Read the model definition and answer for the solid it produces. Units are mm, in the model's axes. Round coordinates to 2 decimals unless told otherwise and drop trailing zeros. Order: outer loops, then holes, each group sorted by start corner. A loop starts at its lowest first (then second) coordinate and runs counter-clockwise, first axis right, second up. Notation, with made-up numbers: (73, 83) - (118, 83) arc R17 ccw to (118, 116) - close; hole circle Ø1 at (43, 25). An arc over 180 degrees is marked (long way). Answer as a JSON object with one key per item and string values. Group by question number.
Q1. Consider line 1 (Y direction, x = 62, z = 1.05); line 2 (X direction, y = -14.75, z = 1.15); line 3 (Y direction, x = 254, z = 0.2). Determine where each line is inside the solid, lowest interval first.
Q2. Given pin 1 Ø4.5 at (x, y) = (254, -13) entering from +Z, flat-ended and moving along its own axis, determine where the tip first touches the part or whether it passes through.
Q3. A cutting plane is placed at A-A on x = 187.5. Determine the outline of the cut face in (y, z) (3 decimals), and give its area (3 significant figures).
Q4. A cutting plane is placed at B-B on z = 1.55. Count the separate pieces of the cut face and the enclosed holes in it, and give its area (3 significant figures).
Autodesk Fusion 360 part; units mm, degrees
sketch "Sketch1" plane through (0, 0, 0) normal (0, 0, 1) x (1, 0, 0)
  line L0 (0, 0) -> (0, -12.7)
  line L1 (12.7, 0) -> (254, 0)
  line L2 (254, -25.4) -> (12.7, -25.4)
  line L3 (0, -25.4) -> (0, -12.7)
  arc A0 (12.7, 0) -> (0, -12.7) centre (12.7, -12.7) ccw
  arc A1 (0, -12.7) -> (12.7, -25.4) centre (12.7, -12.7) ccw
  circle A2 centre (254, -12.7) radius 1.27
  line L4 (254, -25.4) -> (255.27, -25.4)
  line L5 (255.27, 0) -> (254, 0)
  line L6 (255.27, 0) -> (245.11, 0)
  line L7 (245.11, -25.4) -> (255.27, -25.4)
  arc A3 (257.81, -12.7) -> (245.11, 0) centre (245.11, -12.7) ccw
  arc A4 (245.11, -25.4) -> (257.81, -12.7) centre (245.11, -12.7) ccw
  arc A5 (245.11, -19.05) -> (251.46, -12.7) centre (245.11, -12.7) ccw
  arc A6 (251.46, -12.7) -> (245.11, -6.35) centre (245.11, -12.7) ccw
  line L8 (254, -19.05) -> (12.7, -19.05)
  line L9 (12.7, -6.35) -> (254, -6.35)
  arc A7 (12.7, -6.35) -> (6.35, -12.7) centre (12.7, -12.7) ccw
  arc A8 (6.35, -12.7) -> (12.7, -19.05) centre (12.7, -12.7) ccw
  point P0 (0, -25.4)
  point P1 (257.81, 0)
  dimension "d1" = 25.4
  dimension "d3" = 12.7
  dimension "d4" = 12.7
  dimension "d5" = 2.54
  dimension "d6" = 2.54
  dimension "d7" = 12.7
  dimension "d8" = 12.7
  dimension "d9" = -6.35
  dimension "d10" = 6.35
  dimension "d11" = 6.35
  dimension "d12" = -6.35
extrude "Extrude1" add sketch "Sketch1" along normal blind 3.175
sketch "Sketch2" plane through (0, 0, 3.175) normal (0, 0, 1) x (-1, 0, 0)
  circle A0 centre (-254, 12.7) radius 1.27
  arc A1 (-12.7, 6.35) -> (-12.7, 19.05) centre (-12.7, 12.7) ccw
  line L0 (-12.7, 6.35) -> (-245.11, 6.35)
  arc A2 (-245.11, 19.05) -> (-245.11, 6.35) centre (-245.11, 12.7) ccw
  line L1 (-245.11, 19.05) -> (-12.7, 19.05)
  arc A3 (-12.7, 0) -> (-12.7, 25.4) centre (-12.7, 12.7) ccw
  line L2 (-12.7, 25.4) -> (-245.11, 25.4)
  arc A4 (-245.11, 25.4) -> (-245.11, 0) centre (-245.11, 12.7) ccw
  line L3 (-245.11, 0) -> (-12.7, 0)
  circle A5 centre (-254, 12.7) radius 2.0476
extrude "Extrude2" cut sketch "Sketch2" against normal blind 2.54 contours A5
sketch "Sketch3" plane through (0, 0, 3.175) normal (0, 0, 1) x (-1, 0, 0)
  circle A0 centre (-254, 12.7) radius 2.0476
  arc A1 (-12.7, 6.35) -> (-12.7, 19.05) centre (-12.7, 12.7) ccw
  line L0 (-12.7, 6.35) -> (-245.11, 6.35)
  line L1 (-245.11, 19.05) -> (-12.7, 19.05)
  arc A2 (-12.7, 0) -> (-12.7, 25.4) centre (-12.7, 12.7) ccw
  line L2 (-12.7, 25.4) -> (-245.11, 25.4)
  arc A3 (-245.11, 25.4) -> (-245.11, 0) centre (-245.11, 12.7) ccw
  line L3 (-245.11, 0) -> (-12.7, 0)
  line L4 (-245.11, 6.35) -> (-251.46, 6.35)
  line L5 (-251.46, 6.35) -> (-251.46, 19.05)
  line L6 (-251.46, 19.05) -> (-245.11, 19.05)
  line L7 (-245.11, 19.05) -> (-245.11, 6.35)
extrude "Extrude3" add sketch "Sketch3" against normal blind 3.175 contours L4 L5 L6 L7
sketch "Sketch4" plane through (0, 0, 3.175) normal (0, 0, 1) x (-1, 0, 0)
  arc A0 (-12.7, 0) -> (-12.7, 25.4) centre (-12.7, 12.7) ccw
  line L0 (-12.7, 25.4) -> (-245.11, 25.4)
  arc A1 (-245.11, 25.4) -> (-245.11, 0) centre (-245.11, 12.7) ccw
  line L1 (-245.11, 0) -> (-12.7, 0)
  circle A2 centre (-254, 12.7) radius 2.0476
  line L2 (-245.11, 19.05) -> (-12.7, 19.05)
  arc A3 (-12.7, 6.35) -> (-12.7, 19.05) centre (-12.7, 12.7) ccw
  line L3 (-12.7, 6.35) -> (-245.11, 6.35)
  line L4 (-245.11, 6.35) -> (-245.11, 19.05)
  line L5 (-245.11, 0) -> (-260.3587, 0)
  line L6 (-260.3587, 0) -> (-260.3587, 25.4)
  line L7 (-260.3587, 25.4) -> (-245.11, 25.4)
  line L8 (-245.11, 25.4) -> (-245.11, 0)
extrude "Extrude4" add sketch "Sketch4" against normal blind 3.175 contours A1 L5 L6 L7
extrude "Extrude5" cut 1 faces at (254.0316, -14.4834, 0.635) along direction (0, 0, -1) blind 0.3175
draft "Draft1" angle 40 neutral plane through (0, 0, 0.3175) pull (0, 0, 1) 1 faces at (253.949, -14.747, 2.2225)
fillet "Fillet1" radius 12.7 1 edges at (260.3587, -25.4, 1.5875)
fillet "Fillet2" radius 12.7 1 edges at (260.3587, 0, 1.5875)
sketch "Sketch5" plane through (0, 0, 3.175) normal (0, 0, 1) x (-1, 0, 0)
  arc A0 (-247.6587, 25.4) -> (-247.6587, 0) centre (-247.6587, 12.7) ccw
  line L0 (-247.6587, 0) -> (-12.7, 0)
  arc A1 (-12.7, 0) -> (-12.7, 25.4) centre (-12.7, 12.7) ccw
  line L1 (-12.7, 25.4) -> (-247.6587, 25.4)
  line L2 (-245.11, 19.05) -> (-12.7, 19.05)
  arc A2 (-12.7, 6.35) -> (-12.7, 19.05) centre (-12.7, 12.7) ccw
  line L3 (-12.7, 6.35) -> (-245.11, 6.35)
  line L4 (-245.11, 6.35) -> (-245.11, 19.05)
  circle A3 centre (-254, 12.7) radius 4.4453
  line L5 (0, 12.7) -> (-6.35, 12.7)
  line L6 (-0.1678, 12.7) -> (-1.016, 11.938)
  line L7 (-1.016, 11.938) -> (-1.988, 11.0648)
  line L8 (-0.1678, 12.7) -> (-1.016, 13.462)
  line L9 (-1.016, 13.462) -> (-1.988, 14.3352)
  line L10 (-1.988, 11.0648) -> (-1.988, 14.3352)
extrude "Extrude6" cut sketch "Sketch5" against normal blind 0.508 contours L5 L6 L7 L10 | L5 L8 L9 L10
equation "d21 = ( -0.025 / 2 ) * 1 in"
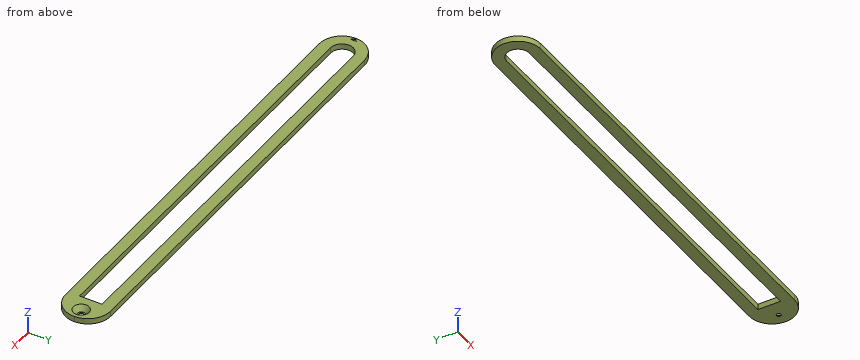
Result set:
{
 "1": {"line 1": "y = -25.4 to -19.05, -6.35 to 0", "line 2": "x = 0.17 to 6.69, 245.11 to 252.17, 255.83 to 260.19", "line 3": "y = -23.7 to -13.97, -11.43 to -1.7"},
 "2": {"pin 1": "stops at z = 0.92"},
 "3": {"outline": "(-25.4, 0) - (-19.05, 0) - (-19.05, 3.175) - (-25.4, 3.175) - close; (-6.35, 0) - (0, 0) - (0, 3.175) - (-6.35, 3.175) - close", "area": "40.3 mm²"},
 "4": {"separate pieces": "1", "enclosed holes": "2", "area": "3,430 mm²"}
}
